```python
from build123d import *

# Parameters (mm, degrees)
SKETCH_W      = 111
SKETCH_H      = 22
PAD_DEPTH     = 3
PAD001_DEPTH  = 3
SKETCH002_W   = 111
SKETCH002_H   = 22
SKETCH002_W_2 = 95.5
SKETCH002_H_2 = 3
PAD002_DEPTH  = 3


with BuildPart() as part:
    # Sketch → Pad (new body)
    with BuildSketch(Plane.XY):
        Rectangle(SKETCH_W, SKETCH_H)
    extrude(amount=PAD_DEPTH)

    # Sketch001 (on Face6 of Pad) → Pad001 (join)
    with BuildSketch(Plane.XY.offset(3)):
        Polygon((-55.5, 11), (55.5, 11), (55.5, 4), (50, 4), (50, 5), (-50, 5), (-50, 4), (-55.5, 4), align=None)
        Polygon((-55.5, -11), (55.5, -11), (55.5, -4), (50, -4), (50, -5), (-50, -5), (-50, -4), (-55.5, -4), align=None)
    extrude(amount=PAD001_DEPTH)

    # Sketch002 (on Face12 of Pad001) → Pad002 (join)
    with BuildSketch(Plane.XY.offset(6)):
        Rectangle(SKETCH002_W, SKETCH002_H)
        Rectangle(SKETCH002_W_2, SKETCH002_H_2, mode=Mode.SUBTRACT)
    extrude(amount=PAD002_DEPTH)


solid = part.part
```
Part model, mm, in its own coordinate system. A direction names the side the tool comes from. Coordinates: 2 decimals unless noted, no trailing zeros. Order: outer loops, then holes, each group sorted by start corner. A loop starts at its lowest first (then second) coordinate and runs counter-clockwise, first axis right, second up. Notation, with made-up numbers: (29.5, -3.5) -> (86.5, -3.5) arc R32 ccw to (86.5, 22.5) -> close; hole circle Ø5 at (0, 53). An arc over 180 degrees is marked (long way). Put each result on its own line as item: value. Start each with the question number.
(1) Probe line 1 along Z through (x, y) = (-48, 4.25); line 2 along Y through (x, z) = (-47, 5.75); line 3 along Y through (x, z) = (40.5, 6.5). List the from-to ranges inside material, lowest first. Write a range as [from, to].
(2) Which spindle directions (+Z, -Z, +X, -X, +Y, -Y) get a long thin tool onto all of the face, cutting with end or side? Do faces 1 (the face through (-1, 0, 3)), 2 (the face through (-53, 4, 4)), 3 (the face through (-1, 1.5, 7)). Say none if no direction does.
(3) Band-saw the part on C-C (x = -7). Give the cut face in (y, z), then the cut area to 3 significant figures.
(4) Mould opens along Z. For faces 4 (the face through (-1, 0, 0)), 5 (the face through (-1, 3, 9)), 6 (the face through (-1, 11, 4)), 7 (the face through (1, 5, 4)) say: pulls with the +Z half, pulls with the -Z half, needs draft (parallel to the pull), parting line crosses it, or undercut.
(5) Band-saw the part on D-D (z = 8). Give the cut face in (x, y), then the cut area to 3 significant figures.
(6) Band-saw the part on B-B (y = 2.75). Give the cut face in (x, z), then the cut area to 3 significant figures.
(7) Band-saw the part on A-A (z = 4). Give the cut face in (x, y), then the cut area to 3 significant figures.
Determined:
1. line 1: z = [0, 3], [6, 9]
1. line 2: y = [-11, -5], [5, 11]
1. line 3: y = [-11, -1.5], [1.5, 11]
2. face 1: none
2. face 2: +X, -X
2. face 3: +Z
3. outline: (-11, 0) -> (11, 0) -> (11, 9) -> (1.5, 9) -> (1.5, 6) -> (5, 6) -> (5, 3) -> (-5, 3) -> (-5, 6) -> (-1.5, 6) -> (-1.5, 9) -> (-11, 9) -> close
3. area: 159 mm²
4. face 4: pulls with the -Z half
4. face 5: pulls with the +Z half
4. face 6: needs draft
4. face 7: undercut
5. outline: (-55.5, -11) -> (55.5, -11) -> (55.5, 11) -> (-55.5, 11) -> close; hole (-47.75, -1.5) -> (47.75, -1.5) -> (47.75, 1.5) -> (-47.75, 1.5) -> close
5. area: 2,160 mm²
6. outline: (-55.5, 0) -> (55.5, 0) -> (55.5, 3) -> (-55.5, 3) -> close; (-55.5, 6) -> (55.5, 6) -> (55.5, 9) -> (-55.5, 9) -> close
6. area: 666 mm²
7. outline: (-55.5, -11) -> (55.5, -11) -> (55.5, -4) -> (50, -4) -> (50, -5) -> (-50, -5) -> (-50, -4) -> (-55.5, -4) -> close; (-55.5, 4) -> (-50, 4) -> (-50, 5) -> (50, 5) -> (50, 4) -> (55.5, 4) -> (55.5, 11) -> (-55.5, 11) -> close
7. area: 1,350 mm²
